```python
from build123d import *

# Parameters (mm, degrees)
CASE_2_DEPTH            = 10
INTERNAL_START          = -2
INTERNAL_SLOT_DEPTH     = 3
CUT_EXTRUDE1_DEPTH      = 83.840207629
CUT_EXTRUDE1_DEPTH_BACK = 83.840207629
SKETCH3_R               = 2


with BuildPart() as part:
    # Sketch1 → Case 2 (new body)
    with BuildSketch(Plane(origin=(0, 0, 0), x_dir=(0, 1, 0), z_dir=(0, 0, 1))):
        with BuildLine():
            Line((-60, -45.5), (60, -45.5))
            ThreePointArc((60, -45.5), (66.01040764, -43.01040764), (68.5, -37))
            Line((68.5, -37), (68.5, 37))
            ThreePointArc((68.5, 37), (66.01040764, 43.01040764), (60, 45.5))
            Line((60, 45.5), (-60, 45.5))
            ThreePointArc((-60, 45.5), (-66.01040764, 43.01040764), (-68.5, 37))
            Line((-68.5, 37), (-68.5, -37))
            ThreePointArc((-68.5, -37), (-66.01040764, -43.01040764), (-60, -45.5))
        make_face()
    extrude(amount=CASE_2_DEPTH)

    # Sketch2 → internal slot (cut)
    with BuildSketch(Plane.XY.offset(10).offset(INTERNAL_START)):
        with BuildLine():
            Line((-37, -62), (37, -62))
            ThreePointArc((37, -62), (38.414213562, -61.414213562), (39, -60))
            Line((39, -60), (39, 60))
            ThreePointArc((39, 60), (38.414213562, 61.414213562), (37, 62))
            Line((37, 62), (-37, 62))
            ThreePointArc((-37, 62), (-38.414213562, 61.414213562), (-39, 60))
            Line((-39, 60), (-39, -60))
            ThreePointArc((-39, -60), (-38.414213562, -61.414213562), (-37, -62))
        make_face()
    extrude(amount=-INTERNAL_SLOT_DEPTH, mode=Mode.SUBTRACT)

    # Sketch3 → Cut-Extrude1 (cut, two sides: drawn at the far end of the back side and taken through both)
    with BuildSketch(Plane.XY.offset(10).offset(-CUT_EXTRUDE1_DEPTH_BACK)):
        with Locations((-40.712310601, 63.712310601)):
            Circle(SKETCH3_R)
        with Locations(Location((-40.712310601, -63.712310601, 0), (0, 0, 180))):
            Circle(SKETCH3_R)
        with Locations(Location((40.712310601, 63.712310601, 0), (0, 0, 180))):
            Circle(SKETCH3_R)
        with Locations((40.712310601, -63.712310601)):
            Circle(SKETCH3_R)
    extrude(amount=CUT_EXTRUDE1_DEPTH + CUT_EXTRUDE1_DEPTH_BACK, mode=Mode.SUBTRACT)


solid = part.part
```
Build history of the part. All positions in model axes, mm. A direction names the side the tool comes from. Round coordinates to 2 decimals unless told otherwise and drop trailing zeros. Write each loop counter-clockwise with the first axis right and the second up, starting at its lowest first coordinate (ties: lowest second). Pieces come first, ordered by that corner, then holes.
1) Mould opens along Z. For faces 3 (the flat face through (-1, 1, 5)), 4 (the cylindrical face through (42.3, 64.93, 4.93)), 5 (the flat face through (-1, -1, 0)) say: +Z half, -Z half, draft (parallel to the pull), parting line (faces both ways), or undercut.
2) 3-axis set-ups, long thin cutter, end or side, ignore diameter. For faces 1 (the flat face through (-1, 1, 8)), 2 (the cylindrical face through (40.279, -65.665, 4.93)): which of +Z, -Z, +X, -X, +Y, -Y reach the whole face in a straight line?
3) Band-saw the part on A-A, the plane x = 7. List the corners of the cut face in (y, z), and give its area (3 significant figures).
4) Band-saw the part on B-B, the plane y = -7. List the corners of the cut face in (x, z), and give its area (3 significant figures).
5) Drill centre lines: probe 1 along X at (y, z) = (-22, 7); probe 2 along Z at (x, y) = (-38, -32.5); probe 3 along Y at (x, z) = (-7.5, 5.25). Where is each one in solid material? Low to high.
Ans:
1. face 3: undercut
1. face 4: draft
1. face 5: -Z half
2. face 1: none
2. face 2: +Z, -Z
3. outline: (-68.5, 0) - (68.5, 0) - (68.5, 10) - (-68.5, 10) - close; hole (-62, 5) - (62, 5) - (62, 8) - (-62, 8) - close
3. area: 998 mm2
4. outline: (-45.5, 0) - (45.5, 0) - (45.5, 10) - (-45.5, 10) - close; hole (-39, 5) - (39, 5) - (39, 8) - (-39, 8) - close
4. area: 676 mm2
5. probe 1: x = -45.5 to -39, 39 to 45.5
5. probe 2: z = 0 to 5, 8 to 10
5. probe 3: y = -68.5 to -62, 62 to 68.5
